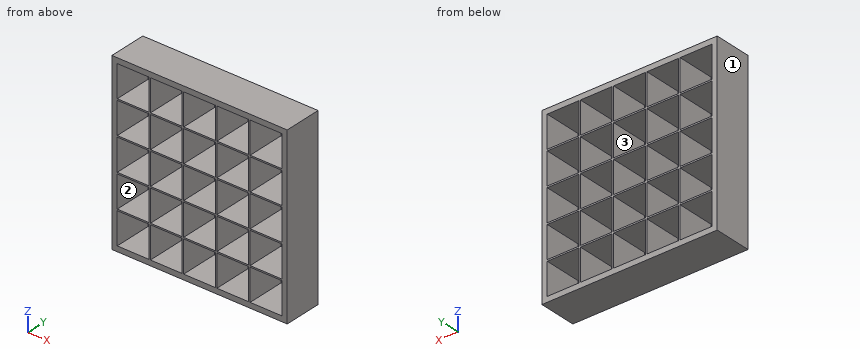
```python
from build123d import *

# Parameters (mm, degrees)
F0_W     = 1820
F0_H     = 1820
F1_DEPTH = 390
F2_W     = 330
F2_H     = 330
F3_DEPTH = 740.61349


with BuildPart() as f1:
    # F0 (on Front) → F1 (new body)
    with BuildSketch(Plane.XZ):
        with Locations((910, 910)):
            Rectangle(F0_W, F0_H)
    extrude(amount=F1_DEPTH)

    # F2 (on Front) → F3 (cut)
    with BuildSketch(Plane.XZ):
        with Locations((220, 220)):
            Rectangle(F2_W, F2_H)
        with Locations((220, 565)):
            Rectangle(F2_W, F2_H)
        with Locations((220, 910)):
            Rectangle(F2_W, F2_H)
        with Locations((220, 1255)):
            Rectangle(F2_W, F2_H)
        with Locations((220, 1600)):
            Rectangle(F2_W, F2_H)
        with Locations((565, 220)):
            Rectangle(F2_W, F2_H)
        with Locations((565, 565)):
            Rectangle(F2_W, F2_H)
        with Locations((565, 910)):
            Rectangle(F2_W, F2_H)
        with Locations((565, 1255)):
            Rectangle(F2_W, F2_H)
        with Locations((565, 1600)):
            Rectangle(F2_W, F2_H)
        with Locations((910, 220)):
            Rectangle(F2_W, F2_H)
        with Locations((910, 565)):
            Rectangle(F2_W, F2_H)
        with Locations((910, 910)):
            Rectangle(F2_W, F2_H)
        with Locations((910, 1255)):
            Rectangle(F2_W, F2_H)
        with Locations((910, 1600)):
            Rectangle(F2_W, F2_H)
        with Locations((1255, 220)):
            Rectangle(F2_W, F2_H)
        with Locations((1255, 565)):
            Rectangle(F2_W, F2_H)
        with Locations((1255, 910)):
            Rectangle(F2_W, F2_H)
        with Locations((1255, 1255)):
            Rectangle(F2_W, F2_H)
        with Locations((1255, 1600)):
            Rectangle(F2_W, F2_H)
        with Locations((1600, 220)):
            Rectangle(F2_W, F2_H)
        with Locations((1600, 565)):
            Rectangle(F2_W, F2_H)
        with Locations((1600, 910)):
            Rectangle(F2_W, F2_H)
        with Locations((1600, 1255)):
            Rectangle(F2_W, F2_H)
        with Locations((1600, 1600)):
            Rectangle(F2_W, F2_H)
    extrude(amount=F3_DEPTH, mode=Mode.SUBTRACT)


solid = f1.part
```
Here's how the part is built. I have some questions about the finished solid (model axes, mm). Face numbers are marked on the shaded views. Give positions to 0.01 mm unless a question says otherwise; leave off trailing zeros. Loops run counter-clockwise (first coordinate to the right, second up) from the corner with the lowest first, then second, coordinate; pieces in that order, holes last. Notation, with made-up numbers: M 39,73.25 L 71,73.25 A33 cw 71,109.25 Z; hole C 6,-39.75 d1. An arc over 180 degrees is marked long. Put each result on its own line as item: value. Start each with the question number.
(1) If we mould it in two halves opening along Z, with no side actions, what happens to the marked faces 1, 2 and 3? For each: +Z half, -Z half, draft (parallel to the pull), parting line (faces both ways), or undercut.
(2) I need wall thicknesses on line 1 along X through (y, z) = (-172.5, 1653). Which ranges of the line are inside material? Lowest first, please. Write a range as [from, to].
(3) I want a section at B-B on z = 1574.5. Please give me the cut outline in (x, y).
(4) I want a section at C-C on y = -316. State how many separate pieces and enclosed holes the cut face has, then the cut area to 3 significant figures.
(5) I want a section at A-A on x = 271. Please give me the cut outline in (y, z).
Answer block:
1. face 1: draft
1. face 2: undercut
1. face 3: undercut
2. line 1: [0, 55], [385, 400], [730, 745], [1075, 1090], [1420, 1435], [1765, 1820]
3. outline: M 0,-390 L 55,-390 L 55,0 L 0,0 Z; M 385,-390 L 400,-390 L 400,0 L 385,0 Z; M 730,-390 L 745,-390 L 745,0 L 730,0 Z; M 1075,-390 L 1090,-390 L 1090,0 L 1075,0 Z; M 1420,-390 L 1435,-390 L 1435,0 L 1420,0 Z; M 1765,-390 L 1820,-390 L 1820,0 L 1765,0 Z
4. separate pieces: 1
4. enclosed holes: 25
4. area: 590,000 mm^2
5. outline: M -390,0 L 0,0 L 0,55 L -390,55 Z; M -390,385 L 0,385 L 0,400 L -390,400 Z; M -390,730 L 0,730 L 0,745 L -390,745 Z; M -390,1075 L 0,1075 L 0,1090 L -390,1090 Z; M -390,1420 L 0,1420 L 0,1435 L -390,1435 Z; M -390,1765 L 0,1765 L 0,1820 L -390,1820 Z
